from build123d import *

# Parameters (mm, degrees)
AUFSATZ_LINEAR_AUSTRAGEN1_DEPTH = 2.8
SCHNITT_LINEAR_START            = 1.5
SKIZZE2_W                       = 3
SKIZZE2_H                       = 2
SCHNITT_LINEAR_AUSTRAGEN1_DEPTH = 2.3
M2_GEWINDEBOHRUNG1_D            = 1.6


with BuildPart() as part:
    # Skizze1 → Aufsatz-Linear austragen1 (new body, symmetric)
    with BuildSketch(Plane.XY):
        Polygon((-9.8, -2), (-1.5, -2), (-1.5, 0), (1.5, 0), (1.5, -2), (9.8, -2), (9.8, -2.5), (5.5, -2.5), (5.5, -9.5), (-5.5, -9.5), (-5.5, -2.5), (-9.8, -2.5), align=None)
    extrude(amount=AUFSATZ_LINEAR_AUSTRAGEN1_DEPTH, both=True)

    # Skizze2 → Schnitt-Linear austragen1 (cut, through all)
    with BuildSketch(Plane.XY.offset(SCHNITT_LINEAR_START)):
        with Locations((0, -1)):
            Rectangle(SKIZZE2_W, SKIZZE2_H)
    schnitt_linear_austragen1 = extrude(amount=SCHNITT_LINEAR_AUSTRAGEN1_DEPTH, mode=Mode.SUBTRACT)

    # Spiegeln1: Schnitt-Linear austragen1 across plane
    add(schnitt_linear_austragen1.mirror(Plane.XY), mode=Mode.SUBTRACT)

    # M2 Gewindebohrung1 (through all)
    with Locations(Plane(origin=(0, -2, 0), x_dir=(1, 0, 0), z_dir=(0, 1, 0))):
        with Locations((-7.5, 0), (7.5, 0)):
            Hole(M2_GEWINDEBOHRUNG1_D / 2)


solid = part.part
Input: part model. Units: mm. Frame: model coordinates. A direction names the side the tool comes from. Round coordinates to 2 decimals unless told otherwise and drop trailing zeros. Write each loop counter-clockwise with the first axis right and the second up, starting at its lowest first coordinate (ties: lowest second). Pieces come first, ordered by that corner, then holes.
1) Contact query for flat-ended pins moving along their axis: P1, Ø1.5, axis at y = -8.5, z = -2, coming from the -X side; P2, Ø3, axis at x = 0.5, z = 0.5, coming from the +Y side; P3, Ø3, axis at y = -7.5, z = 1, coming from the +X side; P4, Ø0.6, axis at x = 0.5, y = -0.5, coming from the -Z side. Output: stop coordinate, or through.
2) Ray query, L1, parallel to Z at x = -7.5, y = -2.2; L2, parallel to X at y = -5.75, z = -1.6; L3, parallel to Y at x = 0, z = -1.7. Return the intervals inside material, ascending.
3) Cut plane D-D (y = -3.5). Return the cut outline in (x, z), then the cut area to 3 significant figures.
4) Draft query along Z for faces 5 (the cylindrical face through (8.3, -2.3, 0)), 6 (the cylindrical face through (-6.7, -2.3, 0)), 7 (the flat face through (0, 0, 0)), 8 (the flat face through (0, -1, 1.5)). Return one class per face: pulls with the +Z half, pulls with the -Z half, needs draft (parallel to the pull), parting line crosses it, or undercut.
5) Reachability of faces 1 (the flat face through (0, -1, -1.5)), 2 (the flat face through (-1.5, -1, 0)), 3 (the flat face through (1.5, -1, 0)), 4 (the flat face through (5.5, -6, 0)) from +Z, -Z, +X, -X, +Y, -Y: full face, straight path, thin tool, end or side. Return the list, or none.
6) Cut plane B-B (x = -7.5). Return the cut outline in (y, z), then the cut area to 3 significant figures.
7) Cut plane C-C (z = -2.35). Return the cut outline in (x, y), then the cut area to 3 significant figures.
8) Cut plane A-A (z = 0). Return the cut outline in (x, y).
Geometry says:
1. P1: stops at x = -5.5
1. P2: stops at y = 0
1. P3: stops at x = 5.5
1. P4: stops at z = -1.5
2. L1: z = -2.8 to -0.8, 0.8 to 2.8
2. L2: x = -5.5 to 5.5
2. L3: y = -9.5 to -2
3. outline: (-5.5, -2.8) - (5.5, -2.8) - (5.5, 2.8) - (-5.5, 2.8) - close
3. area: 61.6 mm2
4. face 5: undercut
4. face 6: undercut
4. face 7: needs draft
4. face 8: pulls with the +Z half
5. face 1: -Z, +X, -X, +Y
5. face 2: +Z, -Z, -X, +Y
5. face 3: +Z, -Z, +X, +Y
5. face 4: +Z, -Z, +X, -Y
6. outline: (-2.5, -2.8) - (-2, -2.8) - (-2, -0.8) - (-2.5, -0.8) - close; (-2.5, 0.8) - (-2, 0.8) - (-2, 2.8) - (-2.5, 2.8) - close
6. area: 2.00 mm2
7. outline: (-9.8, -2.5) - (-5.5, -2.5) - (-5.5, -9.5) - (5.5, -9.5) - (5.5, -2.5) - (9.8, -2.5) - (9.8, -2) - (-9.8, -2) - close
7. area: 86.8 mm2
8. outline: (-9.8, -2.5) - (-8.3, -2.5) - (-8.3, -2) - (-9.8, -2) - close; (-6.7, -2.5) - (-5.5, -2.5) - (-5.5, -9.5) - (5.5, -9.5) - (5.5, -2.5) - (6.7, -2.5) - (6.7, -2) - (1.5, -2) - (1.5, 0) - (-1.5, 0) - (-1.5, -2) - (-6.7, -2) - close; (8.3, -2.5) - (9.8, -2.5) - (9.8, -2) - (8.3, -2) - close
